from build123d import *

# Parameters (mm, degrees)
BOSS_EXTRUDE2_DEPTH = 3


with BuildPart() as part:
    # Sketch1 → Boss-Extrude2 (new body)
    with BuildSketch(Plane(origin=(0, 0, 0), x_dir=(1, 0, 0), z_dir=(0, 1, 0))):
        with BuildLine():
            Line((-60, -10.5), (-60, -90))
            Line((-60, -90), (57, -90))
            Line((57, -90), (57, -30))
            Line((57, -30), (60, -30))
            Line((60, -30), (60, 30))
            Line((60, 30), (57, 30))
            Line((57, 30), (57, 90))
            Line((57, 90), (-60, 90))
            Line((-60, 90), (-60, 10.5))
            ThreePointArc((-60, 10.5), (-49.5, 0), (-60, -10.5))
        make_face()
    extrude(amount=BOSS_EXTRUDE2_DEPTH)


solid = part.part
Can you work these out from the model? Positions are in its coordinate system, mm. Round coordinates to 2 decimals unless told otherwise and drop trailing zeros. Loops run counter-clockwise (first coordinate to the right, second up) from the corner with the lowest first, then second, coordinate; pieces in that order, holes last. Notation, with made-up numbers: (46, 40) - (57, 40) arc R26 ccw to (57, 68) - close; hole circle Ø7 at (63, 89). An arc over 180 degrees is marked (long way). Use CSV: the item, a comma, the result in double quotes. Start each with the question number.
1) Please list where these lines run through material, in increasing order: probe 1 along X at (y, z) = (0.55, 53); probe 2 along Z at (x, y) = (-53, 1.3); probe 3 along Z at (x, y) = (-51.5, 0.5). Write a range as [from, to].
2) For pin 1 Ø4 at (x, z) = (-18.5, -52) entering from -Y; pin 2 Ø0.9 at (x, y) = (58.5, 2) entering from +Z; pin 3 Ø0.9 at (y, z) = (2, -66.5) entering from +X, each with a flat end and sliding along its axis, tell me the tip position at first contact or that it passes through.
3) If we section it at A-A on y = 1.9: Write out the boundary of the cut face in (x, z).
4) If we section it at B-B on z = 0: Write out the boundary of the cut face in (x, y).
5) We'd pull the mould along Y, two halves only. Please class faces 1 (the cylindrical face through (-49.5, 1.5, -0.2)), 2 (the flat face through (-1, 3, -1)), 3 (the flat face through (-1, 0, -1)): released by +Y, released by -Y, zero draft, split by the parting line, or undercut.
Geometry results:
1,probe 1,"x = [-60, 57]"
1,probe 2,"z = [-90, -7.83], [7.83, 90]"
1,probe 3,"z = [-90, -6.16], [6.16, 90]"
2,pin 1,"stops at y = 0"
2,pin 2,"stops at z = 30"
2,pin 3,"stops at x = 57"
3,outline,"(-60, -90) - (57, -90) - (57, -30) - (60, -30) - (60, 30) - (57, 30) - (57, 90) - (-60, 90) - (-60, 10.5) arc R10.5 cw to (-60, -10.5) - close"
4,outline,"(-49.5, 0) - (60, 0) - (60, 3) - (-49.5, 3) - close"
5,face 1,"zero draft"
5,face 2,"released by +Y"
5,face 3,"released by -Y"
